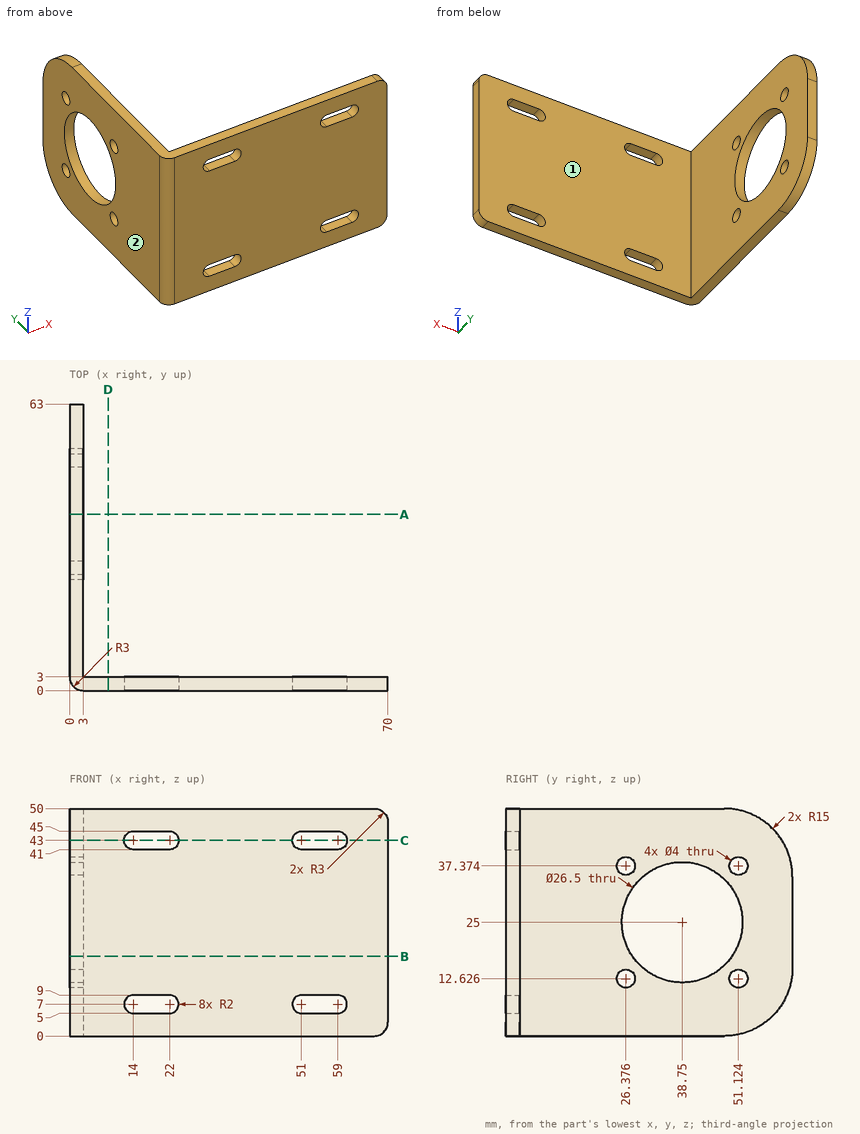
For this review, use the dimensioned drawing (mm, ordinates from the lowest corner) and the shaded views. A direction names the side the tool comes from. Give positions to 0.01 mm unless a question says otherwise; leave off trailing zeros. Write each loop counter-clockwise with the first axis right and the second up, starting at its lowest first coordinate (ties: lowest second). Pieces come first, ordered by that corner, then holes.
(1) Consider section B-B, the plane z = 17.5. Give the boundary of the cut face in (x, y).
(2) Consider section D-D, the plane x = 8.5. Give the boundary of the cut face in (y, z).
(3) For P1, Ø4.5, axis at y = 51.12, z = 37.37, coming from the +X side; P2, Ø2.5, axis at y = 51.12, z = 12.63, coming from the +X side; P3, Ø1, axis at x = 19.5, z = 45, coming from the +Y side, all flat-tipped, find the tip position at first contact; note any pin that passes through.
(4) Consider section A-A, the plane y = 38.75. Give the boundary of the cut face in (x, z), and give its area (3 significant figures).
(5) To check wall thickness, follow L1, parallel to Y at x = 29, z = 7. State the ranges of the line that lie inside material, in increasing order.
(6) Consider section C-C, the plane z = 43. Give the boundary of the cut face in (x, y), and give its area (3 significant figures).
(7) Tool access review of the marked faces 1 and 2: name each direction out of +Z, -Z, +X, -X, +Y, -Y from which nothing blocks a thin tool from reaching the whole face with its end or side.
Returned:
1. outline: (0, 3) arc R3 ccw to (3, 0) - (70, 0) - (70, 3) - (3, 3) - (3, 27.83) - (0, 27.83) - close; (0, 49.67) - (3, 49.67) - (3, 63) - (0, 63) - close
2. outline: (0, 0) - (3, 0) - (3, 50) - (0, 50) - close
3. P1: stops at x = 3
3. P2: passes through
3. P3: stops at y = 3
4. outline: (0, 0) - (3, 0) - (3, 11.75) - (0, 11.75) - close; (0, 38.25) - (3, 38.25) - (3, 50) - (0, 50) - close
4. area: 70.5 mm2
5. L1: y = 0 to 3
6. outline: (0, 3) arc R3 ccw to (3, 0) - (12, 0) - (12, 3) - (3, 3) - (3, 60.69) - (0, 60.69) - close; (24, 0) - (49, 0) - (49, 3) - (24, 3) - close; (61, 0) - (70, 0) - (70, 3) - (61, 3) - close
6. area: 309 mm2
7. face 1: +Z, -Z, +X, +Y
7. face 2: +Z, -Z, -X, +Y, -Y
